For this review, take the finished solid that the model builds, in its own axes (mm). A direction names the side the tool comes from. Give positions to 0.01 mm unless a question says otherwise; leave off trailing zeros. Write each loop counter-clockwise with the first axis right and the second up, starting at its lowest first coordinate (ties: lowest second). Pieces come first, ordered by that corner, then holes. Notation, with made-up numbers: M -33.5,43 L 8.5,43 A24 ccw 8.5,58 Z; hole C -6.75,-2 d10. An arc over 180 degrees is marked long. Use one line per item in the form item = value. Start each with the question number.
Q1. Consider section A-A on x = 19.5. Write out the cut boundary in (y, z), and give its area (3 significant figures).
Q2. Clearance check with a flat-ended pin moving along its axis: pin 1 Ø1.5 at (y, z) = (129, -0.5) entering from -X. State where the tip first meets the part, or that it passes through.
Q3. Tool access review of faces 1 (the flat face through (25, 140, 0)), 2 (the flat face through (21.31, 140.04, -1.48)), 3 (the flat face through (30.464, 138.91, -1.479)): name each direction out of +Z, -Z, +X, -X, +Y, -Y from which nothing blocks a thin tool from reaching the whole face with its end or side.
Q4. Mouldability with a two-part tool opening along Y and no side actions: class faces 4 (the flat face through (25, 140, -3)), 5 (the cylindrical face through (17.9, 214.59, -1.48)) as released by +Y, released by -Y, zero draft, split by the parting line, or undercut.
Q5. Consider section D-D on y = 165.5. Write out the cut boundary in (x, z), and give its area (3 significant figures).
Q6. Consider section C-C on x = 31. Write out the cut boundary in (y, z).
Q7. For probe 1 along X at (y, z) = (90, -0.6); probe 2 along X at (y, z) = (148.5, -1.45); probe 3 along Y at (x, z) = (13, -0.35), list the stretches that pass through material, from the lowest coordinate up. Write a range as [from, to].
Q8. Consider section B-B on z = -1.85. Write out the cut boundary in (x, y).
```python
from build123d import *

# Parameters (mm, degrees)
BOSS_EXTRUDE1_DEPTH = 3


with BuildPart() as part:
    # Sketch1 → Boss-Extrude1 (new body)
    with BuildSketch(Plane.XY):
        with BuildLine():
            ThreePointArc((27.040784053, 219.089006289), (13.163562513, 226.652914674), (14.326848487, 210.891038089))
            Line((14.326848487, 210.891038089), (13.562475801, 218.647695514))
            ThreePointArc((13.562475801, 218.647695514), (17.599473278, 223.567314541), (22.519092305, 219.530317065))
            Line((22.519092305, 219.530317065), (23.28346499, 211.773659641))
            ThreePointArc((23.28346499, 211.773659641), (26.046535999, 214.977080246), (27.040784053, 219.089006289))
        make_face()
        with BuildLine():
            Line((13.562475801, 218.647695514), (14.326848487, 210.891038089))
            ThreePointArc((14.326848487, 210.891038089), (18.923405604, 210.132389785), (23.28346499, 211.773659641))
            Line((23.28346499, 211.773659641), (22.519092305, 219.530317065))
            ThreePointArc((22.519092305, 219.530317065), (18.482094829, 214.610698037), (13.562475801, 218.647695514))
        make_face()
        with BuildLine():
            Line((14.326848487, 210.891038089), (28.489152913, 67.175615091))
            ThreePointArc((28.489152913, 67.175615091), (32.849212299, 68.816884946), (37.445769417, 68.058236642))
            Line((37.445769417, 68.058236642), (23.28346499, 211.773659641))
            ThreePointArc((23.28346499, 211.773659641), (18.923405604, 210.132389785), (14.326848487, 210.891038089))
        make_face()
        with BuildLine():
            ThreePointArc((38.210142102, 60.301579218), (34.173144626, 55.381960191), (29.253525599, 59.418957667))
            Line((29.253525599, 59.418957667), (28.489152913, 67.175615091))
            ThreePointArc((28.489152913, 67.175615091), (29.619907807, 51.854516497), (42.73183385, 59.860268443))
            ThreePointArc((42.73183385, 59.860268443), (41.295742235, 64.737489982), (37.445769417, 68.058236642))
            Line((37.445769417, 68.058236642), (38.210142102, 60.301579218))
        make_face()
        with BuildLine():
            Line((28.489152913, 67.175615091), (29.253525599, 59.418957667))
            ThreePointArc((29.253525599, 59.418957667), (33.290523075, 64.338576695), (38.210142102, 60.301579218))
            Line((38.210142102, 60.301579218), (37.445769417, 68.058236642))
            ThreePointArc((37.445769417, 68.058236642), (32.849212299, 68.816884946), (28.489152913, 67.175615091))
        make_face()
    extrude(amount=-BOSS_EXTRUDE1_DEPTH)


solid = part.part
```
Working result:
q1.outline = M 158.4,-3 L 214.83,-3 L 214.83,0 L 158.4,0 Z; M 223.35,-3 L 227.97,-3 L 227.97,0 L 223.35,0 Z
q1.area = 183 mm²
q2.pin_1 = 22.32
q3.face_1 = +Z, +X, -X, +Y, -Y
q3.face_2 = +Z, -Z, -X
q3.face_3 = +Z, -Z, +X
q4.face_4 = zero draft
q4.face_5 = undercut
q5.outline = M 18.8,-3 L 27.84,-3 L 27.84,0 L 18.8,0 Z
q5.area = 27.1 mm²
q6.outline = M 51.28,-3 L 56.28,-3 L 56.28,0 L 51.28,0 Z; M 63.44,-3 L 133.47,-3 L 133.47,0 L 63.44,0 Z
q7.probe_1 = [26.24, 35.28]
q7.probe_2 = [20.48, 29.52]
q7.probe_3 = [211.63, 226.54]
q8.outline = M 14.33,210.89 L 28.49,67.18 A9 ccw long 37.45,68.06 L 23.28,211.77 A9 ccw long Z; hole C 18.04,219.09 d9; hole C 33.73,59.86 d9
